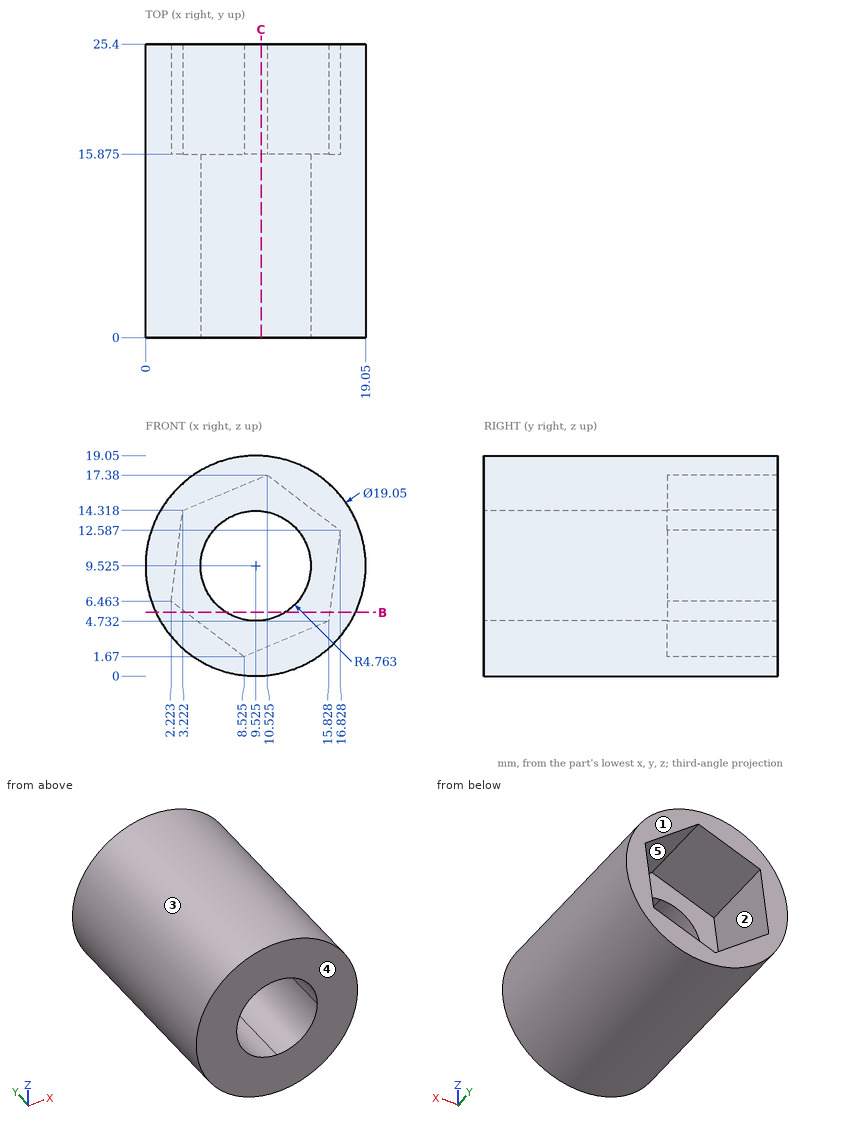
Study the drawing (mm; zero at the part's minimum x, y, z) and answer. A direction names the side the tool comes from. Round coordinates to 2 decimals unless told otherwise and drop trailing zeros. Write each loop counter-clockwise with the first axis right and the second up, starting at its lowest first coordinate (ties: lowest second). Pieces come first, ordered by that corner, then holes. Notation, with made-up numbers: (22, 76.25) -> (73, 76.25) arc R29 cw to (73, 102.25) -> close; hole circle Ø3 at (8.5, 3). An arc over 180 degrees is marked (long way). Answer as CSV lines item,"result". Start each with the question number.
(1) A tool of negligible diameter and unlimited length cuts with its end or side. For the marked faces 4 and 5, from which of +Z, -Z, +X, -X, +Y, -Y can it reach the whole face along a straight path? Write none if from no direction.
(2) The mould has two halves that part along X. Classify the marked faces 1, 2 and 3: +X half, -X half, draft (parallel to the pull), parting line (faces both ways), or undercut.
(3) Each of these flat-tipped pins is pushed along its axis until it touches: pin 1 (1 mm diameter, centred on x = 17, y = 15.5, fed in from +Z); pin 2 (3 mm diameter, centred on x = 7, y = 18, fed in from +Z) (1 decimal); pin 3 (5 mm diameter, centred on y = 15.5, z = 13, fed in from -X). Where does it stop, or does it pass through?
(4) The part is cut by section C-C, the plane x = 10. Give the vertices of the cut face in (y, z) (1 decimal).
(5) The part is cut by section B-B, the plane z = 5.5. Give the vertices of the cut face in (x, y) (1 decimal), then the cut area to 3 significant figures.
(6) Find the intervals of material crossed by probe 1 along Y at (x, z) = (5, 14.75) (1 decimal); probe 2 along X at (y, z) = (12.25, 5.5) (1 decimal); probe 3 along X at (y, z) = (15.25, 7.75) (1 decimal), in increasing order.
Output values:
1,face 4,"+Z, -Z, +X, -X, -Y"
1,face 5,"+Y"
2,face 1,"draft"
2,face 2,"undercut"
2,face 3,"parting line"
3,pin 1,"stops at z = 16.01"
3,pin 2,"stops at z = 19"
3,pin 3,"stops at x = 0.05"
4,outline,"(0, 0) -> (25.4, 0) -> (25.4, 2.3) -> (15.9, 2.3) -> (15.9, 4.8) -> (0, 4.8) -> close; (0, 14.3) -> (15.9, 14.3) -> (15.9, 17.2) -> (25.4, 17.2) -> (25.4, 19) -> (0, 19) -> close"
5,outline,"(0.9, 0) -> (7, 0) -> (7, 15.9) -> (3.5, 15.9) -> (3.5, 25.4) -> (0.9, 25.4) -> close; (12.1, 0) -> (18.2, 0) -> (18.2, 25.4) -> (15.9, 25.4) -> (15.9, 15.9) -> (12.1, 15.9) -> close"
5,area,"239 mm²"
6,probe 1,"y = 0 to 15.9"
6,probe 2,"x = 0.9 to 7, 12.1 to 18.2"
6,probe 3,"x = 0.2 to 5.1, 13.9 to 18.9"
